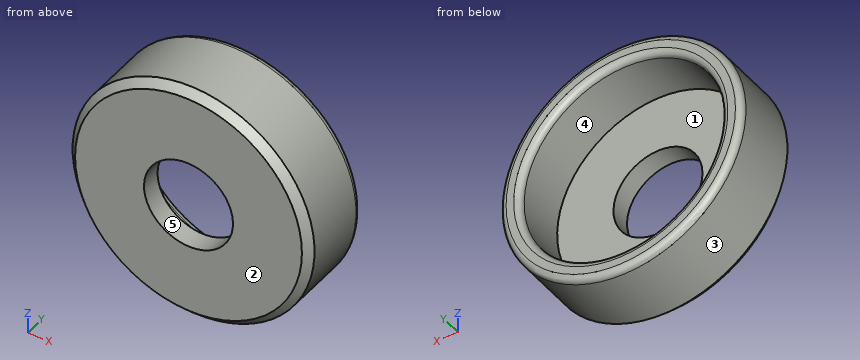
```python
from build123d import *

# Parameters (mm, degrees)
SKETCH2_R          = 1.765
CUT_EXTRUDE1_DEPTH = 8.13582511
FILLET1_R          = 0.25
CHAMFER1_SIZE      = 0.3


with BuildPart() as part:
    # Sketch1 → Revolve1 (revolve)
    with BuildSketch(Plane.XY, mode=Mode.PRIVATE) as revolve1_sk:
        Polygon((0, 0), (4.8, 0), (4.8, 3), (4, 3), (4, 0.8), (0, 0.8), align=None)
    revolve(revolve1_sk.sketch.rotate(Axis((0, 0.8, 0), (0, -1, 0)), 90), axis=Axis((0, 0.8, 0), (0, -1, 0)))

    # Sketch2 → Cut-Extrude1 (cut, through all)
    with BuildSketch(Plane(origin=(0, 0.8, 0), x_dir=(1, 0, 0), z_dir=(0, 1, 0))):
        with Locations(Location((0, 0, 0), (0, 0, 270))):
            Circle(SKETCH2_R)
    extrude(amount=-CUT_EXTRUDE1_DEPTH, mode=Mode.SUBTRACT)

    # Fillet1
    fillet1_edges = [part.edges().sort_by_distance(p)[0] for p in [
        (0, 3, -4),
        (0, 3, -4.8),
    ]]
    fillet(fillet1_edges, radius=FILLET1_R)

    # Chamfer1
    chamfer1_edges = [part.edges().sort_by_distance(p)[0] for p in [
        (0, 0, -4.8),
    ]]
    chamfer(chamfer1_edges, length=CHAMFER1_SIZE)


solid = part.part
```
The model under review builds one solid part; all positions refer to its coordinate system, in mm. Face numbers are marked on the shaded views. A direction names the side the tool comes from. Give positions to 0.01 mm unless a question says otherwise; leave off trailing zeros. Write each loop counter-clockwise with the first axis right and the second up, starting at its lowest first coordinate (ties: lowest second). Pieces come first, ordered by that corner, then holes. Notation, with made-up numbers: M 25,67 L 38,67 A21 ccw 38,81 Z; hole C -2.75,64.5 d8. An arc over 180 degrees is marked long. Answer in a Markdown table with one row per item.
Item 1: Tool access review of the marked faces 4 and 5: name each direction out of +Z, -Z, +X, -X, +Y, -Y from which nothing blocks a thin tool from reaching the whole face with its end or side.
Check sheet entries:
| item | result |
|---|---|
| face 4 | +Y |
| face 5 | +Y, -Y |
Item 2: For line 1 along X through (y, z) = (1.35, 0); line 2 along Y through (x, z) = (2, 0.75); line 3 along Z through (x, y) = (2, 1), list the stretches that pass through material, from the lowest coordinate up.
Check sheet entries:
| item | result |
|---|---|
| line 1 | -4.8 to -4, 4 to 4.8 |
| line 2 | 0 to 0.8 |
| line 3 | -4.36 to -3.46, 3.46 to 4.36 |
Item 3: For P1, Ø2.5, axis at x = -0.5, z = 0.5, coming from the +Y side; P2, Ø1.5, axis at y = 2, z = 3, coming from the +X side, all flat-tipped, find the tip position at first contact; note any pin that passes through.
Check sheet entries:
| item | result |
|---|---|
| P1 | y = 0.8 |
| P2 | x = 4.24 |
Item 4: Add section A-A on x = 0. Give the boundary of the cut face in (y, z) (3 decimals).
Check sheet entries:
| item | result |
|---|---|
| outline | M 0,-4.5 L 0.3,-4.8 L 2.75,-4.8 A0.25 ccw 3,-4.55 L 3,-4.25 A0.25 ccw 2.75,-4 L 0.8,-4 L 0.8,-1.765 L 0,-1.765 Z; M 0,1.765 L 0.8,1.765 L 0.8,4 L 2.75,4 A0.25 ccw 3,4.25 L 3,4.55 A0.25 ccw 2.75,4.8 L 0.3,4.8 L 0,4.5 Z |
Item 5: Draft analysis for pull direction X (two halves, no side actions). For the marked faces 1, 2 and 3, state which applies: +X half, -X half, draft (parallel to the pull), parting line (faces both ways), or undercut.
Check sheet entries:
| item | result |
|---|---|
| face 1 | undercut |
| face 2 | draft |
| face 3 | parting line |
Item 6: Add section C-C on y = 1.8. Give the boundary of the cut face in (x, z), plus the area to 3 significant figures.
Check sheet entries:
| item | result |
|---|---|
| outline | C 0,0 d9.6; hole C 0,0 d8 |
| area | 22.1 mm2 |
Item 7: Add section B-B on z = 0. Give the boundary of the cut face in (x, y) (3 decimals), plus the area to 3 significant figures.
Check sheet entries:
| item | result |
|---|---|
| outline | M -4.8,0.3 L -4.5,0 L -1.765,0 L -1.765,0.8 L -4,0.8 L -4,2.75 A0.25 ccw -4.25,3 L -4.55,3 A0.25 ccw -4.8,2.75 Z; M 1.765,0 L 4.5,0 L 4.8,0.3 L 4.8,2.75 A0.25 ccw 4.55,3 L 4.25,3 A0.25 ccw 4,2.75 L 4,0.8 L 1.765,0.8 Z |
| area | 8.23 mm2 |
